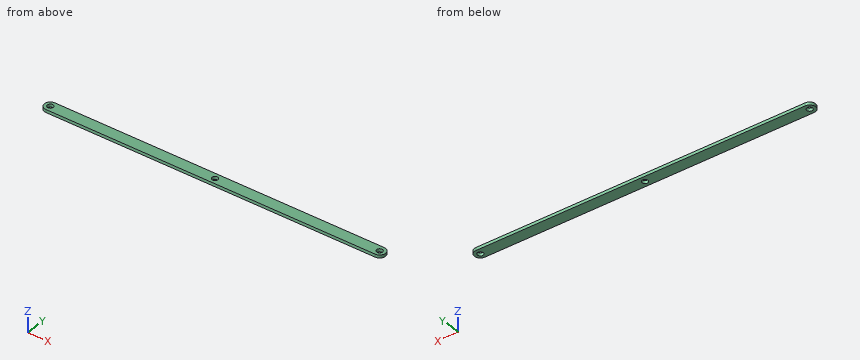
Solid Edge part; units mm, degrees
sketch "Sketch1" plane through (0, 0, 0) normal (0, 0, 1) x (1, 0, 0)
  arc A0 (-282.5, -10) -> (-282.5, 10) centre (-282.5, 0) cw
  line L0 (-282.5, 10) -> (282.5, 10)
  arc A1 (282.5, 10) -> (282.5, -10) centre (282.5, 0) cw
  line L1 (282.5, -10) -> (-282.5, -10)
  circle A2 centre (-282.5, 0) radius 5
  circle A3 centre (282.5, 0) radius 5
  circle A4 centre (0, 0) radius 5
  dimension "D1" = 282.5
  dimension "D2" = 282.5
extrude "Protrusion1" add sketch "Sketch1" against normal blind 5
properties material "Stainless steel"
Geometry check sheet. Reference: the model listing, model coordinates, mm. Give positions to 0.01 mm unless a question says otherwise; leave off trailing zeros. Order: outer loops, then holes, each group sorted by start corner. A loop starts at its lowest first (then second) coordinate and runs counter-clockwise, first axis right, second up.
1) Cross-section at C-C (y = 0). Record the boundary of the cut face in (x, z), then the cut area to 4 significant figures.
Results are:
outline: (-292.5, -5) - (-287.5, -5) - (-287.5, 0) - (-292.5, 0) - close; (-277.5, -5) - (-5, -5) - (-5, 0) - (-277.5, 0) - close; (5, -5) - (277.5, -5) - (277.5, 0) - (5, 0) - close; (287.5, -5) - (292.5, -5) - (292.5, 0) - (287.5, 0) - close
area: 2,775 mm2
2) Gauge pin test, flat end, axial feed: pin 1 (1 mm diameter, centred on y = 4.5, z = -0.5, fed in from +X). Record the tip position at first contact, or that the pin passes through.
Results are:
pin 1: stops at x = 291.67
3) Cross-section at A-A (x = 0). Record the boundary of the cut face in (y, z).
Results are:
outline: (-10, -5) - (-5, -5) - (-5, 0) - (-10, 0) - close; (5, -5) - (10, -5) - (10, 0) - (5, 0) - close
4) Material ranges on probe 1 along Y at (x, z) = (0, -1.3); probe 2 along X at (y, z) = (4.5, -4.6); probe 3 along X at (y, z) = (1.25, -2.9), recorded low to high.
Results are:
probe 1: y = -10 to -5, 5 to 10
probe 2: x = -291.43 to -284.68, -280.32 to -2.18, 2.18 to 280.32, 284.68 to 291.43
probe 3: x = -292.42 to -287.34, -277.66 to -4.84, 4.84 to 277.66, 287.34 to 292.42
5) Cross-section at B-B (z = -3.35). Record the boundary of the cut face in (x, y).
Results are:
outline: (-282.5, -10) - (282.5, -10) arc R10 ccw to (282.5, 10) - (-282.5, 10) arc R10 ccw to start; hole circle Ø10 at (-282.5, 0); hole circle Ø10 at (0, 0); hole circle Ø10 at (282.5, 0)
